```python
from build123d import *

# Parameters (mm, degrees)
EXTRUDE_1_DEPTH        = 13
SKETCH_2_R             = 1.5
SKETCH_2_R_2           = 1.3
CUT_EXTRUDE_1_DEPTH    = 43
CHAMFER_1_SIZE2        = 3
CHAMFER_1_SIZE         = 3.784471042
CHAMFER_1_EDGE_2_SIZE2 = 3
CHAMFER_1_EDGE_2_SIZE  = 3.784471042
CHAMFER_1_EDGE_3_SIZE2 = 3
CHAMFER_1_EDGE_3_SIZE  = 2.56157214
CHAMFER_1_EDGE_4_SIZE2 = 2.56157214
CHAMFER_1_EDGE_4_SIZE  = 3
CHAMFER_2_SIZE         = 2
SKETCH_5_R             = 1.8
EXTRUDE_2_DEPTH        = 3
SKETCH_6_R             = 1.8
CUT_EXTRUDE_2_DEPTH    = 3
SKETCH_7_W             = 3
SKETCH_7_H             = 6.007931748
EXTRUDE_3_DEPTH        = 5.3
SKETCH_8_W             = 1
SKETCH_8_H             = 10
EXTRUDE_4_DEPTH        = 9.5


with BuildPart() as part:
    # 草图1 → 凸台-拉伸1 (new body)
    with BuildSketch(Plane(origin=(0, 0, 0), x_dir=(1, 0, 0), z_dir=(0, 1, 0))):
        Polygon((13, -15.05), (5, -15.05), (5, -11), (-3.5, -11), (-3.5, 11), (5, 11), (5, 15.05), (13, 15.05), (13, 17.05), (5, 17.05), (5, 21), (-5, 21), (-5, 13), (-13, 13), (-13, 10), (-5, 10), (-5, -10), (-13, -10), (-13, -13), (-5, -13), (-5, -21), (5, -21), (5, -17.05), (13, -17.05), align=None)
    extrude(amount=EXTRUDE_1_DEPTH)

    # 草图2 → 切除-拉伸1 (cut, through all)
    with BuildSketch(Plane.XY.offset(21)):
        with Locations((10, 5)):
            Circle(SKETCH_2_R)
        with Locations((-8, 2.5)):
            Circle(SKETCH_2_R)
        with Locations((3.5, 7)):
            Circle(SKETCH_2_R_2)
        Polygon((-13, 7.989732885), (13, 13), (-13, 13), align=None)
    extrude(amount=-CUT_EXTRUDE_1_DEPTH, mode=Mode.SUBTRACT)

    # 倒角1
    chamfer_1_edges = [part.edges().sort_by_distance(p)[0] for p in [
        (-13, 7.989732885, -11.5),
    ]]
    chamfer(chamfer_1_edges, length=CHAMFER_1_SIZE, length2=CHAMFER_1_SIZE2)

    # 倒角1 edge 2
    chamfer_1_edge_2_edges = [part.edges().sort_by_distance(p)[0] for p in [
        (-13, 7.989732885, 11.5),
    ]]
    chamfer(chamfer_1_edge_2_edges, length=CHAMFER_1_EDGE_2_SIZE, length2=CHAMFER_1_EDGE_2_SIZE2)

    # 倒角1 edge 3
    chamfer_1_edge_3_edges = [part.edges().sort_by_distance(p)[0] for p in [
        (13, 13, 16.05),
    ]]
    chamfer(chamfer_1_edge_3_edges, length=CHAMFER_1_EDGE_3_SIZE, length2=CHAMFER_1_EDGE_3_SIZE2)

    # 倒角1 edge 4
    chamfer_1_edge_4_edges = [part.edges().sort_by_distance(p)[0] for p in [
        (13, 13, -16.05),
    ]]
    chamfer(chamfer_1_edge_4_edges, length=CHAMFER_1_EDGE_4_SIZE, length2=CHAMFER_1_EDGE_4_SIZE2)

    # 倒角2
    chamfer_2_edges = [part.edges().sort_by_distance(p)[0] for p in [
        (0, 10.494866442, -21),
        (0.75, 10.639393378, 11),
        (0.75, 10.639393378, -11),
        (0, 10.494866442, 21),
    ]]
    chamfer(chamfer_2_edges, length=CHAMFER_2_SIZE)

    # 草图5 → 凸台-拉伸2 (add)
    with BuildSketch(Plane(origin=(-3.5, 0, 0), x_dir=(0, 0, -1), z_dir=(1, 0, 0))):
        Polygon((0, 10.468681012), (-3.003965874, 8.734340506), (-3.003965874, 5.265659494), (0, 3.531318988), (3.003965874, 5.265659494), (3.003965874, 8.734340506), align=None)
        with Locations((0, 7)):
            Circle(SKETCH_5_R, mode=Mode.SUBTRACT)
    extrude(amount=EXTRUDE_2_DEPTH)

    # 草图6 → 切除-拉伸2 (cut)
    with BuildSketch(Plane(origin=(-3.5, 0, 0), x_dir=(0, 0, -1), z_dir=(1, 0, 0))):
        with Locations((0, 7)):
            Circle(SKETCH_6_R)
    extrude(amount=-CUT_EXTRUDE_2_DEPTH, mode=Mode.SUBTRACT)

    # 草图7 → 凸台-拉伸3 (add)
    with BuildSketch(Plane.XZ):
        with Locations((-2, 0)):
            Rectangle(SKETCH_7_W, SKETCH_7_H)
    extrude(amount=-EXTRUDE_3_DEPTH)

    # 草图8 → 凸台-拉伸4 (add)
    with BuildSketch(Plane.XZ):
        with Locations((5.5, 16)):
            Rectangle(SKETCH_8_W, SKETCH_8_H)
        with Locations((5.5, -16)):
            Rectangle(SKETCH_8_W, SKETCH_8_H)
    extrude(amount=-EXTRUDE_4_DEPTH)


solid = part.part
```
Check sheet for the modelled part. Datum: model origin and axes. Units: mm. A direction names the side the tool comes from. Give positions to 0.01 mm unless a question says otherwise; leave off trailing zeros. Loops run counter-clockwise (first coordinate to the right, second up) from the corner with the lowest first, then second, coordinate; pieces in that order, holes last. Notation, with made-up numbers: M 18.25,89.5 L 63.25,89.5 A22 cw 63.25,111.5 Z; hole C 2,56.25 d5. An arc over 180 degrees is marked long. Answer as CSV lines item,"result".
Item 1: Sectioned sample at A-A, the plane z = 18.5. Enter the section's corners in (x, y).
Reply:
outline,"M -5,0 L 6,0 L 6,9.5 L 5,9.5 L 5,11.46 L -5,9.53 Z; hole C 3.5,7 d2.6"
Item 2: Draft check along Y on faces 1 (the face through (8.5, 5.07, -16.04)), 2 (the face through (4.1, 5.847, 16.07)), 3 (the face through (-13, 2, -12)), 4 (the face through (5.5, 9.5, 19.1)). Enter one of: pulls with the +Y half, pulls with the -Y half, needs draft (parallel to the pull), parting line crosses it, or undercut.
Reply:
face 1,"undercut"
face 2,"undercut"
face 3,"needs draft"
face 4,"pulls with the +Y half"
Item 3: Sectioned sample at B-B, the plane x = 3.5. Enter the section's corners in (y, z), then the cut area to 3 significant figures.
Reply:
outline,"M 0,-21 L 5.7,-21 L 5.7,-11 L 0,-11 Z; M 0,11 L 5.7,11 L 5.7,21 L 0,21 Z; M 8.3,-21 L 9.13,-21 L 11.17,-19 L 11.17,-13 L 9.13,-11 L 8.3,-11 Z; M 8.3,11 L 9.13,11 L 11.17,13 L 11.17,19 L 9.13,21 L 8.3,21 Z"
area,"163 mm^2"
Item 4: Depth check by flat-ended pin: pin 1 Ø4 at (y, z) = (3, -18) entering from -X; pin 2 Ø5 at (x, y) = (10, 5) entering from +Z; pin 3 Ø10 at (x, z) = (-8.5, -8.5) entering from -Y; pin 4 Ø1.1 at (x, z) = (5.5, -18.5) entering from +Y. Enter the tip coordinate at first touch or a pass-through.
Reply:
pin 1,"x = -5"
pin 2,"z = 17.05"
pin 3,"y = 0"
pin 4,"y = 11.46"
Item 5: Sectioned sample at C-C, the plane y = 2.5. State how many separate pieces and enclosed holes the cut face has, then the cut area to 3 significant figures.
Reply:
separate pieces,"3"
enclosed holes,"0"
area,"329 mm^2"
Item 6: Scan lines: L1, parallel to Z at x = -2.85, y = 7; L2, parallel to Z at x = -1.5, y = 4.25; L3, parallel to Z at x = 10.5, y = 12. Record each from-to range of solid material in increasing order.
Reply:
L1,"-21 to -11, -3 to -1.8, 1.8 to 3, 11 to 21"
L2,"-21 to -11, -3 to 3, 11 to 21"
L3,"-17.05 to -15.05, 15.05 to 17.05"
Item 7: Sectioned sample at D-D, the plane x = -8. Enter the section's corners in (y, z).
Reply:
outline,"M 0,-13 L 1,-13 L 1,-10 L 0,-10 Z; M 0,10 L 1,10 L 1,13 L 0,13 Z; M 4,-13 L 8.95,-13 L 8.95,-10 L 4,-10 Z; M 4,10 L 8.95,10 L 8.95,13 L 4,13 Z"
Item 8: Set-up check for faces 5 (the face through (-5, 5, -17)), 6 (the face through (-9, 5, 10)), 7 (the face through (-9, 5, 13)), 8 (the face through (12, 11, 16)), 9 (the face through (5.5, 9.5, -19)): record each of +Z, -Z, +X, -X, +Y, -Y from which the full face is reachable in a straight line by a thin tool's end or side.
Reply:
face 5,"-Z, -X, +Y, -Y"
face 6,"-X, +Y, -Y"
face 7,"+Z, -X, +Y, -Y"
face 8,"+Z, +X, +Y"
face 9,"-Z, +X, +Y"
